Autodesk Inventor part; units mm, degrees
ref_plane "YZ Plane" through (0, 0, 0) normal (1, 0, 0) x (0, 1, 0)
ref_plane "XZ Plane" through (0, 0, 0) normal (0, 1, 0) x (-1, 0, 0)
ref_plane "XY Plane" through (0, 0, 0) normal (0, 0, 1) x (1, 0, 0)
sketch "Sketch1" plane through (0, 0, 0) normal (0, 0, 1) x (1, 0, 0)
  line L0 (-8.8404, 43.5319) -> (-1.8404, 43.5319)
  line L1 (-1.8404, 43.5319) -> (-1.8404, 3.5319)
  line L2 (-1.8404, 3.5319) -> (90.1596, 3.5319)
  line L3 (90.1596, 3.5319) -> (90.1596, -6.4681)
  line L4 (90.1596, -6.4681) -> (-8.8404, -6.4681)
  line L5 (-8.8404, -6.4681) -> (-8.8404, 43.5319)
  point P0 (0, 0)
  dimension "d0" = 10
  dimension "d1" = 50
  dimension "d2" = 7
  dimension "d4" = 92
extrude "Extrusion1" add sketch "Sketch1" along normal blind 45
sketch "Sketch3" plane through (90.1596, -6.4681, 0) normal (1, 0, 0) x (0, 0, -1)
  circle A0 centre (-22.5, 23) radius 19
  line L0 (0, 0) -> (-45, 0)
  line L1 (-45, 0) -> (-45, 10)
  point P0 (0, 6.4681)
  dimension "d7" = 38
  dimension "d8" = 23
  dimension "d9" = 22.5
extrude "Extrusion2" cut sketch "Sketch3" against normal up to surface (92 mm away)
sketch "Sketch4" plane through (-1.8404, 3.5319, 0) normal (1, 0, 0) x (0, 0, -1)
  arc A0 (-36.3564, 0) -> (-8.6436, 0) centre (-22.5, 13) ccw
  circle A1 centre (-22.5, 13) radius 19
  circle A2 centre (-22.5, 6) radius 3.25
  line L0 (0, -10) -> (0, 0)
  circle A3 centre (-22.5, 13) radius 15.5
  circle A4 centre (-38, 13) radius 2.166
  circle A5 centre (-30.25, 26.4234) radius 2.1809
  circle A6 centre (-14.75, 26.4234) radius 2.0998
  circle A7 centre (-7, 13) radius 1.7963
  circle A8 centre (-14.75, -0.4234) radius 2.628
  circle A9 centre (-30.25, -0.4234) radius 2.0573
  line L1 (-38, 13) -> (-22.5, 13)
  line L2 (-22.5, 13) -> (-7, 13)
  line L3 (-14.75, 26.4234) -> (-22.5, 13)
  line L4 (-14.75, -0.4234) -> (-22.5, 13)
  line L5 (-30.25, -0.4234) -> (-22.5, 13)
  line L6 (-30.25, 26.4234) -> (-22.5, 13)
  point P0 (0, -3.5319)
  dimension "d12" = 38
  dimension "d13" = 7
  dimension "d14" = 6.5
  dimension "d15" = 22.5
  dimension "d16" = 31
  dimension "d17" = 60
  dimension "d18" = 60
  dimension "d19" = 60
  dimension "d20" = 60
hole "Hole1" at (-1.8404, 29.9553, 30.25) at (-1.8404, 29.9553, 14.75) at (-1.8404, 16.5319, 7) at (-1.8404, 3.1085, 14.75) at (-1.8404, 3.1085, 30.25) at (-1.8404, 16.5319, 38) direction (-1, 0, 0) diameter 3.3 end through all
sketch "Sketch5" plane through (-1.8404, 3.5319, 0) normal (1, 0, 0) x (0, 0, -1)
  point P0 (0, -3.5319)
sketch "Sketch6" plane through (-1.8404, 3.5319, 0) normal (1, 0, 0) x (0, 0, -1)
  circle A0 centre (-22.5, 6) radius 6
  line L0 (-45, 0) -> (-45, 40)
  arc A1 (-36.3564, 0) -> (-8.6436, 0) centre (-22.5, 13) ccw
  circle A2 centre (-22.5, 13) radius 19
  point P0 (0, -3.5319)
  dimension "d28" = 12
  dimension "d29" = 22.5
  dimension "d30" = 7
extrude "Extrusion3" cut sketch "Sketch6" against normal up to surface (7 mm away) contours A0
sketch "Sketch7" plane through (0, 0, 45) normal (0, 0, 1) x (1, 0, 0)
  line L0 (-8.8404, 43.5319) -> (-8.8404, -6.4681)
  line L1 (91.1596, -6.4681) -> (-8.8404, -6.4681)
  line L2 (-8.8404, -6.4681) -> (-8.8404, -2.4681)
  line L3 (-8.8404, -2.4681) -> (91.1596, -2.4681)
  line L4 (91.1596, -2.4681) -> (91.1596, -6.4681)
  point P0 (90.1596, 3.5319)
  dimension "d33" = 4
  dimension "d55" = 100
extrude "Extrusion4" add sketch "Sketch7" along normal blind 15 and the other way blind 60
sketch "Sketch8" plane through (-8.8404, -2.4681, 0) normal (0, 1, 0) x (1, 0, 0)
  circle A0 centre (10, 7.5) radius 4.4582
  circle A1 centre (90, 7.5) radius 4.9921
  circle A2 centre (10, -52.5) radius 4.3054
  circle A3 centre (90, -52.5) radius 4.5947
  line L0 (0, 15) -> (100, 15)
  line L1 (0, 15) -> (0, 0)
  line L2 (100, 15) -> (100, -60)
  line L3 (100, 15) -> (100, -60)
  line L4 (100, -60) -> (0, -60)
  line L5 (0, -45) -> (0, -60)
  circle A4 centre (50, -52.5) radius 3.4509
  circle A5 centre (50, 7.5) radius 3.4509
  point P0 (8.8404, 0)
  point P1 (99, 0)
  point P2 (99, -45)
  dimension "d38" = 7.5
  dimension "d39" = 10
  dimension "d40" = 10
  dimension "d41" = 7.5
  dimension "d42" = 10
  dimension "d43" = 7.5
  dimension "d44" = 10
  dimension "d45" = 7.5
  dimension "d53" = 50
  dimension "d54" = 50
hole "Hole2" at (1.1596, -2.4681, -7.5) at (81.1596, -2.4681, -7.5) at (81.1596, -2.4681, 52.5) at (1.1596, -2.4681, 52.5) at (41.1596, -2.4681, 52.5) at (41.1596, -2.4681, -7.5) direction (0, -1, 0) diameter 3.3 end through all
properties part number "Support_moteur"
Source: CAD feature listing. Evaluate the final solid. Frame: model axes, mm. A direction names the side the tool comes from. Round coordinates to 2 decimals unless told otherwise and drop trailing zeros. Loops run counter-clockwise (first coordinate to the right, second up) from the corner with the lowest first, then second, coordinate; pieces in that order, holes last. Notation, with made-up numbers: (-15.75, 53) - (18.25, 53) arc R5 cw to (18.25, 59) - close; hole circle Ø3 at (64.25, 57.25). An arc over 180 degrees is marked (long way). Write item = value, one per line. Start each with the question number.
Item 1: Material intervals for line 1 (X direction, y = -4.05, z = -7.5); line 2 (Y direction, x = -6, z = 22); line 3 (Y direction, x = -6, z = 7), sorted ascending.
Item 2: Section query C-C on x = 38. Output: boundary loops of the cut face in (y, z), plus the area to 3 significant figures.
Item 3: Mould query, pull axis Z, two halves, no side actions, for faces 1 (the face through (44, 3.532, 4)), 2 (the face through (40, -4, 60)), 3 (the face through (41.09, -4.5, 50.85)), 4 (the face through (40, -4, -15)). Classes: released by +Z, released by -Z, zero draft, split by the parting line, or undercut.
Item 4: Reachability of faces 5 (the face through (22, 2, 0)), 6 (the face through (44, 3.532, 41)), 7 (the face through (42, -6.468, 22)) from +Z, -Z, +X, -X, +Y, -Y: full face, straight path, thin tool, end or side. Return the list, or none.
Item 5: Section query D-D on y = 6. Output: boundary loops of the cut face in (x, z), plus the area to 3 significant figures.
Item 6: Section query A-A on z = 52.5. Output: boundary loops of the cut face in (x, y).
Item 7: Section query B-B on z = 7. Output: boundary loops of the cut face in (x, y).
Item 8: First-contact query: pin 1 Ø9.5 at (x, z) = (40.5, 4.5) entering from +Y; pin 2 Ø2.5 at (x, z) = (1.16, 52.5) entering from -Y; pin 3 Ø19 at (y, z) = (9.53, 22.5) entering from +X; pin 4 Ø8 at (y, z) = (6, 40.5) entering from +X. Flat tips, straight axial feed; report the tip coordinate or a pass-through.
Results list:
q1.line_1 = -8.84 to -0.49, 2.81 to 39.51, 42.81 to 79.51, 82.81 to 91.16
q1.line_2 = -6.47 to 3.55, 15.51 to 43.53
q1.line_3 = -6.47 to 14.88, 18.18 to 43.53
q2.outline = (-6.47, -15) - (-2.47, -15) - (-2.47, 0) - (3.53, 0) - (3.53, 8.64) arc R19 cw to (3.53, 36.36) - (3.53, 45) - (-2.47, 45) - (-2.47, 60) - (-6.47, 60) - close
q2.area = 455 mm²
q3.face_1 = zero draft
q3.face_2 = released by +Z
q3.face_3 = undercut
q3.face_4 = released by -Z
q4.face_5 = -Z, +X, -X, +Y
q4.face_6 = +Z, -Z, +X, +Y
q4.face_7 = +Z, -Z, +X, -X, -Y
q5.outline = (-8.84, 0) - (-1.84, 0) - (-1.84, 17.65) - (-8.84, 17.65) - close; (-8.84, 27.35) - (-1.84, 27.35) - (-1.84, 45) - (-8.84, 45) - close
q5.area = 247 mm²
q6.outline = (-8.84, -6.47) - (-0.49, -6.47) - (-0.49, -2.47) - (-8.84, -2.47) - close; (2.81, -6.47) - (39.51, -6.47) - (39.51, -2.47) - (2.81, -2.47) - close; (42.81, -6.47) - (79.51, -6.47) - (79.51, -2.47) - (42.81, -2.47) - close; (82.81, -6.47) - (91.16, -6.47) - (91.16, -2.47) - (82.81, -2.47) - close
q7.outline = (-8.84, -6.47) - (91.16, -6.47) - (91.16, -2.47) - (90.16, -2.47) - (90.16, 3.53) - (-1.84, 3.53) - (-1.84, 14.88) - (-8.84, 14.88) - close; (-8.84, 18.18) - (-1.84, 18.18) - (-1.84, 43.53) - (-8.84, 43.53) - close
q8.pin_1 = 3.53
q8.pin_2 = through
q8.pin_3 = -1.84
q8.pin_4 = 90.16
